The listing builds one solid part. Answer for the finished solid, in the listing's coordinates (mm). A direction names the side the tool comes from. Coordinates: 2 decimals unless noted, no trailing zeros. Order: outer loops, then holes, each group sorted by start corner. A loop starts at its lowest first (then second) coordinate and runs counter-clockwise, first axis right, second up. Notation, with made-up numbers: (24.5, -24) -> (56.5, -24) arc R15 ccw to (56.5, -17) -> close; hole circle Ø1 at (-31, -2). An arc over 180 degrees is marked (long way). Return JSON: item names as keys, results as strings.
```python
from build123d import *

# Parameters (mm, degrees)
SKETCH_1_R          = 20
SKETCH_1_R_2        = 1.55
SKETCH_1_R_3        = 2.05
EXTRUDE_1_DEPTH     = 6
SKETCH_2_R          = 12.5
CUT_EXTRUDE_1_DEPTH = 31
CUT_EXTRUDE_2_DEPTH = 1.65
CUT_EXTRUDE_3_DEPTH = 1.65


with BuildPart() as part:
    # 草图1 → 凸台-拉伸1 (new body)
    with BuildSketch(Plane.XY):
        Circle(SKETCH_1_R)
        with Locations((0, 15)):
            Circle(SKETCH_1_R_2, mode=Mode.SUBTRACT)
        with Locations((15, 0)):
            Circle(SKETCH_1_R_2, mode=Mode.SUBTRACT)
        with Locations((0, -15)):
            Circle(SKETCH_1_R_2, mode=Mode.SUBTRACT)
        with Locations((-15, 0)):
            Circle(SKETCH_1_R_2, mode=Mode.SUBTRACT)
        with Locations((-11.313708499, 11.313708499)):
            Circle(SKETCH_1_R_3, mode=Mode.SUBTRACT)
        with Locations((11.313708499, 11.313708499)):
            Circle(SKETCH_1_R_3, mode=Mode.SUBTRACT)
        with Locations((11.313708499, -11.313708499)):
            Circle(SKETCH_1_R_3, mode=Mode.SUBTRACT)
        with Locations((-11.313708499, -11.313708499)):
            Circle(SKETCH_1_R_3, mode=Mode.SUBTRACT)
    extrude(amount=EXTRUDE_1_DEPTH)

    # 草图2 → 切除-拉伸1 (cut)
    with BuildSketch(Plane(origin=(0, 0, 0), x_dir=(-1, 0, 0), z_dir=(0, 0, -1))):
        Circle(SKETCH_2_R)
    extrude(amount=-CUT_EXTRUDE_1_DEPTH, mode=Mode.SUBTRACT)

    # 草图4 → 切除-拉伸2 (cut)
    with BuildSketch(Plane(origin=(0, 0, 0), x_dir=(-1, 0, 0), z_dir=(0, 0, -1))):
        with BuildLine():
            Line((-3.697159098, 19.655304999), (-5.515511779, 11.217358415))
            ThreePointArc((-5.515511779, 11.217358415), (0, 12.5), (5.515511779, 11.217358415))
            Line((5.515511779, 11.217358415), (3.697159098, 19.655304999))
            ThreePointArc((3.697159098, 19.655304999), (0, 20), (-3.697159098, 19.655304999))
        make_face()
        with BuildLine():
            Line((19.655304999, -3.697159098), (11.217358415, -5.515511779))
            ThreePointArc((11.217358415, -5.515511779), (12.5, 0), (11.217358415, 5.515511779))
            Line((11.217358415, 5.515511779), (19.655304999, 3.697159098))
            ThreePointArc((19.655304999, 3.697159098), (20, 0), (19.655304999, -3.697159098))
        make_face()
        with BuildLine():
            Line((-3.697159098, -19.655304999), (-5.515511779, -11.217358415))
            ThreePointArc((-5.515511779, -11.217358415), (0, -12.5), (5.515511779, -11.217358415))
            Line((5.515511779, -11.217358415), (3.697159098, -19.655304999))
            ThreePointArc((3.697159098, -19.655304999), (0, -20), (-3.697159098, -19.655304999))
        make_face()
        with BuildLine():
            Line((-19.655304999, 3.697159098), (-11.217358415, 5.515511779))
            ThreePointArc((-11.217358415, 5.515511779), (-12.5, 0), (-11.217358415, -5.515511779))
            Line((-11.217358415, -5.515511779), (-19.655304999, -3.697159098))
            ThreePointArc((-19.655304999, -3.697159098), (-20, 0), (-19.655304999, 3.697159098))
        make_face()
    extrude(amount=-CUT_EXTRUDE_2_DEPTH, mode=Mode.SUBTRACT)

    # 草图5 → 切除-拉伸3 (cut)
    with BuildSketch(Plane(origin=(0, 0, 0), x_dir=(-1, 0, 0), z_dir=(0, 0, -1))):
        with BuildLine():
            Line((3.697159098, 19.655304999), (5.515511779, 11.217358415))
            ThreePointArc((5.515511779, 11.217358415), (8.838834765, 8.838834765), (11.217358415, 5.515511779))
            Line((11.217358415, 5.515511779), (19.655304999, 3.697159098))
            ThreePointArc((19.655304999, 3.697159098), (14.142135624, 14.142135624), (3.697159098, 19.655304999))
        make_face()
    extrude(amount=-CUT_EXTRUDE_3_DEPTH, mode=Mode.SUBTRACT)


solid = part.part
```
Item 1: Find the intervals of material crossed by probe 1 along Y at (x, z) = (0, 2.55); probe 2 along Y at (x, z) = (1, 2.7), in increasing order.
Answer list:
{"probe 1": "-20 to -16.55, -13.45 to -12.5, 12.5 to 13.45, 16.55 to 20", "probe 2": "-19.97 to -16.18, -13.82 to -12.46, 12.46 to 13.82, 16.18 to 19.97"}
Item 2: Which of the six approach directions +Z, -Z, +X, -X, +Y, -Y give full straight-line access (tool end or side, diameter ignored) to faces 1 (the flat face through (15.38, -4.62, 0.81)), 2 (the flat face through (4.594, 15.495, 0.813)), 3 (the cylindrical face through (9.687, 10.066, 2.958))?
Answer list:
{"face 1": "-Z", "face 2": "-Z, -X", "face 3": "+Z, -Z"}
Item 3: Determine the mould class of faces 4 (the flat face through (-15.495, -4.594, 0.813)), 5 (the flat face through (4.594, -15.495, 0.813)), 6 (the flat face through (13.3, -9.8, 0)) for opening direction Y: pulls with the +Y half, pulls with the -Y half, needs draft (parallel to the pull), parting line crosses it, or undercut.
Answer list:
{"face 4": "pulls with the +Y half", "face 5": "undercut", "face 6": "needs draft"}
Item 4: The part is cut by section D-D on y = -5. Determine the outline of the cut face in (x, z), plus the area to 3 significant figures.
Answer list:
{"outline": "(-19.36, 0) -> (-13.61, 0) -> (-13.61, 1.65) -> (-11.46, 1.65) -> (-11.46, 6) -> (-19.36, 6) -> close; (11.46, 1.65) -> (13.61, 1.65) -> (13.61, 0) -> (19.36, 0) -> (19.36, 6) -> (11.46, 6) -> close", "area": "87.8 mm2"}
Item 5: The part is cut by section A-A on y = 0. Determine the outline of the cut face in (x, z).
Answer list:
{"outline": "(-20, 1.65) -> (-16.55, 1.65) -> (-16.55, 6) -> (-20, 6) -> close; (-13.45, 1.65) -> (-12.5, 1.65) -> (-12.5, 6) -> (-13.45, 6) -> close; (12.5, 1.65) -> (13.45, 1.65) -> (13.45, 6) -> (12.5, 6) -> close; (16.55, 1.65) -> (20, 1.65) -> (20, 6) -> (16.55, 6) -> close"}
Item 6: The part is cut by section C-C on z = 1.1. Determine the outline of the cut face in (x, y), plus the area to 3 significant figures.
Answer list:
{"outline": "(-19.66, -3.7) arc R20 ccw to (-3.7, -19.66) -> (-5.52, -11.22) arc R12.5 cw to (-11.22, -5.52) -> close; (3.7, -19.66) arc R20 ccw to (19.66, -3.7) -> (11.22, -5.52) arc R12.5 cw to (5.52, -11.22) -> close; (3.7, 19.66) -> (5.52, 11.22) arc R12.5 cw to (11.22, 5.52) -> (19.66, 3.7) arc R20 ccw to start; hole circle Ø4.1 at (-11.31, -11.31); hole circle Ø4.1 at (11.31, -11.31); hole circle Ø4.1 at (11.31, 11.31)", "area": "325 mm2"}
Item 7: Flat-ended cylindrical pins translate along their axes: pin 1 (1 mm diameter, centred on x = -5.5, y = 13, fed in from -Z); pin 2 (3 mm diameter, centred on y = -2, z = 1, fed in from +X); pin 3 (1.5 mm diameter, centred on x = -7, z = 2, fed in from -Y). Find the tip coordinate at first contact, or state that the pin passes through.
Answer list:
{"pin 1": "z = 1.65", "pin 2": "x = 19.99", "pin 3": "y = -19"}
